Geometry check sheet. Reference: the model listing, model coordinates, mm. Round coordinates to 2 decimals unless told otherwise and drop trailing zeros. Write each loop counter-clockwise with the first axis right and the second up, starting at its lowest first coordinate (ties: lowest second). Pieces come first, ordered by that corner, then holes. Notation, with made-up numbers: (41.25, 89.25) -> (96.25, 89.25) arc R24 cw to (96.25, 102.25) -> close; hole circle Ø8 at (5, 54.25). An arc over 180 degrees is marked (long way). One line per question, with ' | ' between items.
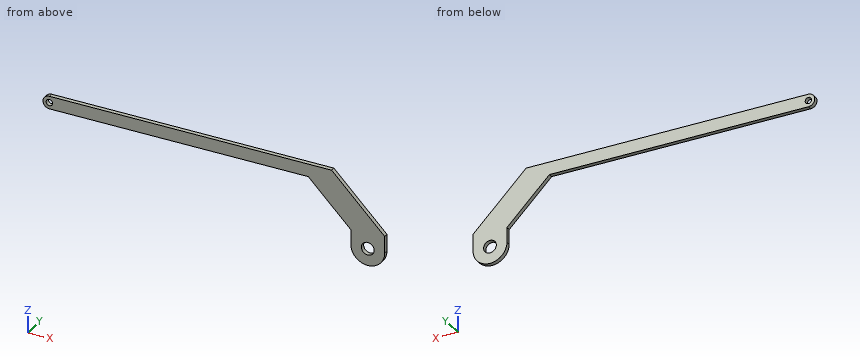
```python
from build123d import *

# Parameters (mm, degrees)
SKETCH1_R           = 1.5
SKETCH1_R_2         = 0.75
BOSS_EXTRUDE1_DEPTH = 1


with BuildPart() as part:
    # Sketch1 → Boss-Extrude1 (new body)
    with BuildSketch(Plane(origin=(0, 0, 0), x_dir=(1, 0, 0), z_dir=(0, 1, 0))):
        with BuildLine():
            Line((-4, 0), (-4, -3.5))
            Line((-4, -3.5), (-14, -13.5))
            Line((-14, -13.5), (-75, -13.5))
            ThreePointArc((-75, -13.5), (-76.5, -15), (-75, -16.5))
            Line((-75, -16.5), (-8.514718626, -16.5))
            Line((-8.514718626, -16.5), (4, -3.985281374))
            Line((4, -3.985281374), (4, 0))
            ThreePointArc((4, 0), (0, 4), (-4, 0))
        make_face()
        with Locations(Location((0, 0, 0), (0, 0, 270))):
            Circle(SKETCH1_R, mode=Mode.SUBTRACT)
        with Locations(Location((-75, -15, 0), (0, 0, 270))):
            Circle(SKETCH1_R_2, mode=Mode.SUBTRACT)
    extrude(amount=BOSS_EXTRUDE1_DEPTH)


solid = part.part
```
(1) Sectioned sample at D-D on z = 2.75. Record the cut outline in (x, y), then the cut area to 3 significant figures.
Resolved:
outline: (-4, 0) -> (4, 0) -> (4, 1) -> (-4, 1) -> close | area: 8.00 mm2
(2) Go/stop test with a flat-tipped pin: pin 1 (1.4 mm diameter, centred on x = -75, z = 15, fed in from -Y). Record where the tip stops, or that it passes through.
Resolved:
pin 1: passes through
(3) Sectioned sample at B-B on z = 15. Record the cut outline in (x, y), then the cut area to 3 significant figures.
Resolved:
outline: (-76.5, 0) -> (-75.75, 0) -> (-75.75, 1) -> (-76.5, 1) -> close; (-74.25, 0) -> (-7.01, 0) -> (-7.01, 1) -> (-74.25, 1) -> close | area: 68.0 mm2
(4) Material ranges on line 1 (X direction, y = 0.35, z = 0); line 2 (X direction, y = 0.6, z = 2.75); line 3 (Z direction, x = -70, y = 0.9), recorded low to high.
Resolved:
line 1: x = -4 to -1.5, 1.5 to 4 | line 2: x = -4 to 4 | line 3: z = 13.5 to 16.5
(5) Sectioned sample at A-A on y = 0.3. Record the cut outline in (x, z).
Resolved:
outline: (-75, 13.5) -> (-14, 13.5) -> (-4, 3.5) -> (-4, 0) arc R4 ccw to (4, 0) -> (4, 3.99) -> (-8.51, 16.5) -> (-75, 16.5) arc R1.5 ccw to start; hole circle Ø1.5 at (-75, 15); hole circle Ø3 at (0, 0)
(6) Sectioned sample at C-C on x = -25.5. Record the cut outline in (y, z), then the cut area to 3 significant figures.
Resolved:
outline: (0, 13.5) -> (1, 13.5) -> (1, 16.5) -> (0, 16.5) -> close | area: 3.00 mm2
